Autodesk Inventor part; units mm, degrees
ref_plane "YZ Plane" through (0, 0, 0) normal (1, 0, 0) x (0, 1, 0)
ref_plane "XZ Plane" through (0, 0, 0) normal (0, 1, 0) x (-1, 0, 0)
ref_plane "XY Plane" through (0, 0, 0) normal (0, 0, 1) x (1, 0, 0)
sketch "Sketch1" plane through (0, 0, 0) normal (0, 1, 0) x (-1, 0, 0)
  line L0 (0, 0) -> (-197.3834, 0)
  line L1 (-197.3834, 0) -> (-197.3834, 84.1502)
  line L2 (-197.3834, 84.1502) -> (-114.3, 165.1)
  line L3 (-114.3, 165.1) -> (-114.3, 222.25)
  line L4 (-114.3, 222.25) -> (0, 222.25)
  line L5 (0, 222.25) -> (0, 0)
  dimension "d9" = 197.3834
  dimension "d10" = 222.25
  dimension "d11" = 84.1502
  dimension "d12" = 114.3
  dimension "d13" = 57.15
extrude "Extrusion1" add sketch "Sketch1" along normal blind 25.4
sketch "Sketch2" plane through (0, 25.4, 0) normal (0, 1, 0) x (1, 0, 0)
  circle A0 centre (12.7, -177.8) radius 12.7
  line L0 (0, -222.25) -> (114.3, -222.25)
  line L1 (0, 0) -> (0, -222.25)
  dimension "d14" = 44.45
  dimension "d15" = 25.4
  dimension "d16" = 12.7
extrude "Extrusion2" add sketch "Sketch2" along normal blind 25.4
properties part number "handmove"
Input: part model. Units: mm. Frame: model coordinates. A direction names the side the tool comes from. Round coordinates to 2 decimals unless told otherwise and drop trailing zeros. Loops run counter-clockwise (first coordinate to the right, second up) from the corner with the lowest first, then second, coordinate; pieces in that order, holes last. Notation, with made-up numbers: (-3.5, 9.25) - (2.5, 9.25) arc R27 ccw to (2.5, 43.25) - close; hole circle Ø9 at (47.25, -19.5). An arc over 180 degrees is marked (long way). One line per item, written item: value. Start each with the question number.
(1) Section B-B, the plane z = 184.5. Return loops of the section in (x, y), plus the area to 3 significant figures.
(2) Section A-A, the plane x = 12.7. Return loops of the section in (y, z).
(3) Ray query, line 1 (Y direction, x = 84, z = 207); line 2 (X direction, y = 8.5, z = 172.5); line 3 (Z direction, x = 163, y = 6). Return the intervals inside material, ascending. Write a range as [from, to].
(4) Contact query for flat-ended pins moving along their axis: P1, Ø5, axis at x = 26, z = 110, coming from the +Y side; P2, Ø12.5, axis at y = 13.5, z = 192.5, coming from the +X side. Output: stop coordinate, or through.
(5) Section D-D, the plane y = 36.5. Return loops of the section in (x, z).
(6) Access query for faces 1 (the cylindrical face through (19.527, 37.922, 188.509)), 2 (the flat face through (114.3, 13, 193)), 3 (the flat face through (13, 50.8, 178)). Directions: +Z, -Z, +X, -X, +Y, -Y. A direction counts if a zero-diameter tool reaches every point of the face in a straight line with its end or side. Return the directions, or none.
(7) Section C-C, the plane y = 19.5. Return loops of the section in (x, z), plus the area to 3 significant figures.
Results below:
1. outline: (0, 0) - (114.3, 0) - (114.3, 25.4) - (23.49, 25.4) - (23.49, 50.8) - (1.91, 50.8) - (1.91, 25.4) - (0, 25.4) - close
1. area: 3,450 mm^2
2. outline: (0, 0) - (25.4, 0) - (25.4, 165.1) - (50.8, 165.1) - (50.8, 190.5) - (25.4, 190.5) - (25.4, 222.25) - (0, 222.25) - close
3. line 1: [0, 25.4]
3. line 2: [0, 114.3]
3. line 3: [0, 117.65]
4. P1: y = 25.4
4. P2: x = 114.3
5. outline: circle Ø25.4 at (12.7, 177.8)
6. face 1: +Y
6. face 2: +Z, +X, +Y, -Y
6. face 3: +Z, -Z, +X, -X, +Y
7. outline: (0, 0) - (197.38, 0) - (197.38, 84.15) - (114.3, 165.1) - (114.3, 222.25) - (0, 222.25) - close
7. area: 35,800 mm^2
